Design review of the part built by this model. Coordinates are the model's own, in mm. Give positions to 0.01 mm unless a question says otherwise; leave off trailing zeros. Order: outer loops, then holes, each group sorted by start corner. A loop starts at its lowest first (then second) coordinate and runs counter-clockwise, first axis right, second up. Notation, with made-up numbers: M -35.75,75.5 L 0.25,75.5 A19 ccw 0.25,103.5 Z; hole C -26.5,-24.5 d4. An arc over 180 degrees is marked long. Answer as a JSON object with one key per item and string values.
Autodesk Inventor part; units mm, degrees
ref_plane "YZ Plane" through (0, 0, 0) normal (1, 0, 0) x (0, 1, 0)
ref_plane "XZ Plane" through (0, 0, 0) normal (0, 1, 0) x (-1, 0, 0)
ref_plane "XY Plane" through (0, 0, 0) normal (0, 0, 1) x (1, 0, 0)
sketch "Sketch1" plane through (0, 0, 0) normal (0, 1, 0) x (-1, 0, 0)
  circle A0 centre (-40, 0) radius 4.5
  circle A1 centre (20, -34.641) radius 4.5
  circle A2 centre (20, 34.641) radius 4.5
  line L0 (40, -23.094) -> (26.6667, -46.188)
  line L1 (26.6667, -46.188) -> (0, -46.188)
  line L2 (-40, -23.094) -> (-53.3333, 0)
  line L3 (-53.3333, 0) -> (-40, 23.094)
  line L4 (0, 46.188) -> (26.6667, 46.188)
  line L5 (26.6667, 46.188) -> (40, 23.094)
  arc A3 (-40, 23.094) -> (0, 46.188) centre (-39.3111, 68.0887) ccw
  arc A4 (0, -46.188) -> (-40, -23.094) centre (-39.3111, -68.0887) ccw
  arc A5 (40, 23.094) -> (40, -23.094) centre (78.6221, 0) ccw
  point P0 (0, 0)
  point P1 (0, 0)
  point P2 (0, 0)
  point P3 (0, 0)
  dimension "d1" = 9
  dimension "d2" = 9
  dimension "d3" = 9
  dimension "d4" = 45
  dimension "d5" = 45
  dimension "d6" = 45
extrude "Extrusion1" add sketch "Sketch1" along normal blind 5
properties part number "Palm1"
(1) We need section D-D (x = 31). Write out the cut boundary in (y, z), plus the area to 3 significant figures.
Checked values:
{"outline": "M 0,-23.86 L 5,-23.86 L 5,23.86 L 0,23.86 Z", "area": "239 mm^2"}
(2) To check wall thickness, follow L1, parallel to Z at x = -20, y = 2.25; L2, parallel to Z at x = 40, y = 2.35; L3, parallel to Z at x = -16.5, y = 2.55. State the ranges of each line that lie inside material, in increasing order. Write a range as from..to.
Checked values:
{"L1": "z = -46.19..-39.14, -30.14..30.14, 39.14..46.19", "L2": "z = -23.09..-4.5, 4.5..23.09", "L3": "z = -46.19..-37.47, -31.81..31.81, 37.47..46.19"}
(3) We need section C-C (y = 3.3). Write out the cut boundary in (x, z).
Checked values:
{"outline": "M -40,-23.09 L -26.67,-46.19 L 0,-46.19 A45 cw 40,-23.09 L 53.33,0 L 40,23.09 A45 cw 0,46.19 L -26.67,46.19 L -40,23.09 A45 cw Z; hole C -20,-34.64 d9; hole C -20,34.64 d9; hole C 40,0 d9"}
(4) Draft analysis for pull direction Z (two halves, no side actions). For faces 1 (the cylindrical face through (17.106, 2.465, -28.949)), 2 (the cylindrical face through (-16.683, 2.465, 31.6)), 3 (the flat face through (-33.24, 2.46, 34.8)), state which applies: +Z half, -Z half, draft (parallel to the pull), parting line (faces both ways), or undercut.
Checked values:
{"face 1": "-Z half", "face 2": "undercut", "face 3": "+Z half"}
(5) Insertion check: pin 1 (3 mm diameter, centred on x = 39.5, y = 3, fed in from -Z); pin 2 (7 mm diameter, centred on x = -20, z = 34.641, fed in from +Y); pin 3 (1 mm diameter, centred on x = 41.5, y = 2.5, fed in from +Z); pin 4 (1.5 mm diameter, centred on x = 19, y = 2.5, fed in from -Z). Each pin has a flat end and moves straight along its axis. Give the tip position at first contact, or say it passes through.
Checked values:
{"pin 1": "stops at z = -23.11", "pin 2": "passes through", "pin 3": "stops at z = 21.36", "pin 4": "stops at z = -28.32"}
(6) We need section A-A (x = -20). Write out the cut boundary in (y, z).
Checked values:
{"outline": "M 0,-46.19 L 5,-46.19 L 5,-39.14 L 0,-39.14 Z; M 0,-30.14 L 5,-30.14 L 5,30.14 L 0,30.14 Z; M 0,39.14 L 5,39.14 L 5,46.19 L 0,46.19 Z"}
(7) We need section B-B (z = 1.5). Write out the cut boundary in (x, y).
Checked values:
{"outline": "M -33.65,0 L 35.76,0 L 35.76,5 L -33.65,5 Z; M 44.24,0 L 52.47,0 L 52.47,5 L 44.24,5 Z"}
